Could you check a few things on this model? Use its own coordinates, in mm. A direction names the side the tool comes from. Give positions to 0.01 mm unless a question says otherwise; leave off trailing zeros. Loops run counter-clockwise (first coordinate to the right, second up) from the corner with the lowest first, then second, coordinate; pieces in that order, holes last.
1. For P1, Ø4, axis at x = 10, z = 4.5, coming from the +Y side, with a flat end and sliding along its axis, tell me the tip position at first contact or that it passes through.
2. For faces 1 (the flat face through (-60.2, 21, 1)), 2 (the flat face through (62, 8, -5)), 3 (the flat face through (63.2, 14, 1)), 4 (the flat face through (60.2, 14, 1)), 5 (the flat face through (-5, 23, 39)), which set-ups out of +Z, -Z, +X, -X, +Y, -Y let a thin tool reach every point of the face, with its end or its side?
3. I need wall thicknesses on line 1 along X through (y, z) = (20.5, 26); line 2 along Z through (x, y) = (45.5, 18.75); line 3 along Z through (x, y) = (-18.5, 8.5). Which ranges of each line are inside material? Lowest first, please.
4. Imagine slicing it at B-B (y = 20.5). List the corners of the cut face in (x, z) for me.
5. Thinking about a two-plate mould opening in Z: for faces 6 (the flat face through (-1, 11, 40.7)), 7 (the flat face through (-1, 21, 37.7)), 8 (the flat face through (57.5, 8, -39)), which applies, +Z half, -Z half, draft (parallel to the pull), parting line (faces both ways), or undercut?
```python
from build123d import *

# Parameters (mm, degrees)
BOSS_EXTRUDE1_DEPTH = 3
SKETCH2_W           = 126.4
SKETCH2_H           = 81.4
SKETCH2_W_2         = 120.4
SKETCH2_H_2         = 75.4
BOSS_EXTRUDE2_DEPTH = 20
SKETCH4_W           = 7.2
SKETCH4_H           = 20
CUT_EXTRUDE1_DEPTH  = 10
SKETCH5_W           = 15
SKETCH5_H           = 12.33485255
CUT_EXTRUDE2_DEPTH  = 10
BOSS_EXTRUDE3_START = -4
SKETCH6_W           = 120.4
SKETCH6_H           = 75.4
SKETCH6_W_2         = 116.4
SKETCH6_H_2         = 71.4
BOSS_EXTRUDE3_DEPTH = 2
CHAMFER1_SIZE       = 2


with BuildPart() as part:
    # Sketch1 → Boss-Extrude1 (new body)
    with BuildSketch(Plane(origin=(0, 0, 0), x_dir=(1, 0, 0), z_dir=(0, 1, 0))):
        Polygon((63.2, 40.7), (-63.2, 40.7), (-63.2, -40.7), (63.2, -40.7), (63.2, -15), (63.2, 5), align=None)
    extrude(amount=BOSS_EXTRUDE1_DEPTH)

    # Sketch2 → Boss-Extrude2 (add)
    with BuildSketch(Plane(origin=(0, 3, 0), x_dir=(1, 0, 0), z_dir=(0, 1, 0))):
        Rectangle(SKETCH2_W, SKETCH2_H)
        Rectangle(SKETCH2_W_2, SKETCH2_H_2, mode=Mode.SUBTRACT)
    extrude(amount=BOSS_EXTRUDE2_DEPTH)

    # Sketch4 → Cut-Extrude1 (cut)
    with BuildSketch(Plane(origin=(0, 3, 0), x_dir=(1, 0, 0), z_dir=(0, 1, 0))):
        with Locations((59.6, -5)):
            Rectangle(SKETCH4_W, SKETCH4_H)
    extrude(amount=CUT_EXTRUDE1_DEPTH, mode=Mode.SUBTRACT)

    # Sketch5 → Cut-Extrude2 (cut)
    with BuildSketch(Plane(origin=(0, 3, 0), x_dir=(1, 0, 0), z_dir=(0, 1, 0))):
        with Locations((50, 37.5)):
            Rectangle(SKETCH5_W, SKETCH5_H)
    extrude(amount=CUT_EXTRUDE2_DEPTH, mode=Mode.SUBTRACT)

    # Sketch6 → Boss-Extrude3 (add)
    with BuildSketch(Plane(origin=(0, 23, 0), x_dir=(1, 0, 0), z_dir=(0, 1, 0)).offset(BOSS_EXTRUDE3_START)):
        Rectangle(SKETCH6_W, SKETCH6_H)
        Rectangle(SKETCH6_W_2, SKETCH6_H_2, mode=Mode.SUBTRACT)
    extrude(amount=-BOSS_EXTRUDE3_DEPTH)

    # Chamfer1
    chamfer1_edges = [part.edges().sort_by_distance(p)[0] for p in [
        (0, 17, 37.7),
        (-60.2, 17, 0),
        (0, 17, -37.7),
        (60.2, 17, 0),
    ]]
    chamfer(chamfer1_edges, length=CHAMFER1_SIZE - 0.0001)  # a hair under: the kernel refuses the full size


solid = part.part
```
Derived:
1. P1: stops at y = 3
2. face 1: +Y
2. face 2: +X
2. face 3: +Z, -Z, +X, +Y, -Y
2. face 4: none
2. face 5: +Z, -Z, +X, -X, +Y
3. line 1: x = -63.2 to -60.2, 60.2 to 63.2
3. line 2: z = -40.7 to -35.7, 35.7 to 40.7
3. line 3: z = -40.7 to -37.7, 37.7 to 40.7
4. outline: (-63.2, -40.7) - (63.2, -40.7) - (63.2, 40.7) - (-63.2, 40.7) - close; hole (-60.2, -37.7) - (60.2, -37.7) - (60.2, 37.7) - (-60.2, 37.7) - close
5. face 6: +Z half
5. face 7: undercut
5. face 8: draft
